Autodesk Fusion 360 part; units mm, degrees
sketch "base" plane through (0, 0, 0) normal (0, 0, 1) x (1, 0, 0)
  line L0 (0, 0) -> (19, 0)
  line L1 (19, 0) -> (19, 44.4)
  line L2 (19, 44.4) -> (0, 44.4)
  line L3 (0, 44.4) -> (0, 0)
  dimension "d1" = 19
  dimension "d2" = 44.4
extrude "Extrude1" add sketch "base" along normal blind 2
sketch "walls" plane through (0, 0, 2) normal (0, 0, 1) x (-1, 0, 0)
  line L0 (0, -44.4) -> (0, 0)
  line L1 (0, 0) -> (-19, 0)
  line L2 (-19, 0) -> (-19, -44.4)
  line L3 (-19, -44.4) -> (0, -44.4)
  line L4 (0, 0) -> (-19, 0)
  line L5 (-19, 0) -> (-19, -44.4)
  line L6 (-19, -44.4) -> (0, -44.4)
  line L7 (0, -44.4) -> (0, 0)
  line L8 (-1.2, -12) -> (-17.8, -12)
  line L9 (-17.8, -12) -> (-17.8, -36.4)
  line L10 (-15.3, -41.2) -> (-3.7, -41.2)
  line L11 (-1.2, -36.4) -> (-1.2, -12)
  line L12 (-1.2, -36.4) -> (-3.7, -41.2)
  line L13 (-17.8, -36.4) -> (-15.3, -41.2)
  dimension "d5" = 19
  dimension "d6" = 44.4
  dimension "d7" = 16.6
  dimension "d9" = 12
  dimension "d10" = 1.2
  dimension "d59" = 4.8
  dimension "d61" = 4.8
  dimension "d62" = 2.5
  dimension "d63" = 11.6
  dimension "d64" = 3.2
  dimension "d71" = 2.5
extrude "Extrude2" add sketch "walls" along normal blind 12
sketch "hole for connector" plane through (0, 0, 0) normal (0, -1, 0) x (1, 0, 0)
  line L0 (0, 0) -> (19, 0)
  line L1 (19, 0) -> (19, 14)
  line L2 (19, 14) -> (0, 14)
  line L3 (0, 14) -> (0, 0)
  line L4 (0, 14) -> (19, 14) construction
  line L5 (19, 14) -> (19, 2) construction
  line L6 (19, 2) -> (0, 2) construction
  line L7 (0, 2) -> (0, 14) construction
  line L8 (9.5, 14) -> (9.5, 0) construction
  line L9 (4.5, 8.4) -> (14.5, 8.4)
  line L10 (14.5, 8.4) -> (14.5, 2)
  line L11 (14.5, 2) -> (4.5, 2)
  line L12 (4.5, 2) -> (4.5, 8.4)
  dimension "d13" = 10
  dimension "d14" = 6.4
  dimension "d15" = 2
  dimension "d16" = 4.5
extrude "Extrude3" cut sketch "hole for connector" against normal blind 7 contours L9 L10 L11 L12
sketch "stand for rare of pcb" plane through (0, 0, 2) normal (0, 0, 1) x (-1, 0, 0)
  line L0 (-1.2, -12) -> (-17.8, -12)
  line L1 (-17.8, -12) -> (-17.8, -36.4)
  line L2 (-15.3, -41.2) -> (-3.7, -41.2)
  line L3 (-1.2, -36.4) -> (-1.2, -12)
  line L4 (-7.7, -41.2) -> (-11.3, -41.2)
  line L5 (-11.3, -41.2) -> (-11.3, -27)
  line L6 (-11.3, -27) -> (-7.7, -27)
  line L7 (-7.7, -27) -> (-7.7, -41.2)
  line L8 (-17.8, -12) -> (-1.2, -12)
  line L9 (-17.8, -36.4) -> (-15.3, -41.2)
  line L10 (-3.7, -41.2) -> (-1.2, -36.4)
  dimension "d27" = 3.6
  dimension "d28" = 15
  dimension "d29" = 6.5
extrude "Extrude5" add sketch "stand for rare of pcb" along normal blind 9 contours L2 L4 L5 L6 L7
sketch "hole for connector pins" plane through (0, 7, 0) normal (0, -1, 0) x (1, 0, 0)
  line L0 (4.5, 2) -> (14.5, 2)
  line L1 (14.5, 2) -> (14.5, 8.4)
  line L2 (14.5, 8.4) -> (4.5, 8.4)
  line L3 (4.5, 8.4) -> (4.5, 2)
  line L4 (5.5, 7.6) -> (13.5, 7.6)
  line L5 (13.5, 7.6) -> (13.5, 2)
  line L6 (13.5, 2) -> (5.5, 2)
  line L7 (5.5, 2) -> (5.5, 7.6)
  dimension "d32" = 8
  dimension "d33" = 5.6
  dimension "d34" = 5.5
  dimension "d35" = 2
extrude "Extrude6" cut sketch "hole for connector pins" against normal blind 5 contours L0 L4 L5 L6 L7
sketch "pit for pcb" plane through (0, 0, 14) normal (0, 0, 1) x (-1, 0, 0)
  line L0 (-1.2, -12) -> (-1.2, -36.4)
  line L1 (-3.7, -41.2) -> (-15.3, -41.2)
  line L2 (-17.8, -36.4) -> (-17.8, -12)
  line L3 (-17.8, -12) -> (-1.2, -12)
  line L4 (0, -44.4) -> (0, 0)
  line L5 (0, 0) -> (-19, 0)
  line L6 (-19, 0) -> (-19, -44.4)
  line L7 (-19, -44.4) -> (0, -44.4)
  line L8 (-2, -12) -> (-17, -12)
  line L9 (-17, -12) -> (-17, -3.2)
  line L10 (-17, -3.2) -> (-2, -3.2)
  line L11 (-2, -3.2) -> (-2, -12)
  line L12 (-1.2, -36.4) -> (-3.7, -41.2)
  line L13 (-15.3, -41.2) -> (-17.8, -36.4)
  dimension "d44" = 15
  dimension "d45" = 8.8
  dimension "d46" = 2
  dimension "d47" = 3.2
extrude "Extrude7" cut sketch "pit for pcb" against normal blind 3 contours L3 L8 L9 L10 L11
fillet "Fillet1" radius 1.5 4 edges at (19, 0, 7) (0, 0, 7) (0, 44.4, 7) (19, 44.4, 7)
sketch "pit for wires" plane through (0, 0, 11) normal (0, 0, 1) x (-1, 0, 0)
  line L0 (-2, -3.2) -> (-17, -3.2)
  line L1 (-17, -3.2) -> (-17, -12)
  line L2 (-2, -12) -> (-2, -3.2)
  line L3 (-4.5, -3.2) -> (-14.5, -3.2)
  line L4 (-14.5, -3.2) -> (-14.5, -7.2)
  line L5 (-4.5, -7.2) -> (-4.5, -3.2)
  line L6 (-2, -12) -> (-17, -12)
  line L7 (-17, -12) -> (-17, -7.2)
  line L8 (-2, -7.2) -> (-2, -12)
  line L9 (-17, -7.2) -> (-14.5, -7.2)
  line L10 (-4.5, -7.2) -> (-2, -7.2)
  line L11 (-17, -12) -> (-2, -12)
  dimension "d48" = 10
  dimension "d49" = 2.5
  dimension "d51" = 4
  dimension "d65" = 2.5
extrude "Extrude8" cut sketch "pit for wires" against normal blind 2 contours L0 L1 L2 L3 L4 L5 L6 L7 L8 L9 L10 L11
sketch "mount cylinder" plane through (0, 0, 11) normal (0, 0, 1) x (-1, 0, 0)
  line L0 (-7.7, -27) -> (-11.3, -27)
  line L1 (-11.3, -27) -> (-11.3, -41.2)
  line L2 (-11.3, -41.2) -> (-7.7, -41.2)
  line L3 (-7.7, -41.2) -> (-7.7, -27)
  circle A0 centre (-9.5, -38.2) radius 1
  line L4 (-17.8, -36.4) -> (-17.8, -12)
  dimension "d54" = 2
  dimension "d55" = 3
  dimension "d56" = 8.3
extrude "Extrude9" add sketch "mount cylinder" along normal blind 3 contours A0
sketch "mount cylinder 2" plane through (0, 0, 9) normal (0, 0, 1) x (-1, 0, 0)
  line L0 (-14.5, -3.2) -> (-14.5, -7.2)
  line L1 (-14.5, -7.2) -> (-17, -7.2)
  line L2 (-17, -7.2) -> (-17, -12)
  line L3 (-17, -12) -> (-2, -12)
  line L4 (-2, -12) -> (-2, -7.2)
  line L5 (-2, -7.2) -> (-4.5, -7.2)
  line L6 (-4.5, -7.2) -> (-4.5, -3.2)
  circle A0 centre (-9.5, -10.2) radius 1
  line L7 (-4.5, -3.2) -> (-14.5, -3.2)
  dimension "d66" = 2
  dimension "d68" = 7.5
  dimension "d72" = 7
extrude "Extrude10" add sketch "mount cylinder 2" along normal blind 3 contours A0
sketch "lock notch front" plane through (0, 0, 0) normal (0, -1, 0) x (1, 0, 0)
  line L0 (14.5, 8.4) -> (14.5, 2)
  line L1 (14.5, 2) -> (4.5, 2)
  line L2 (4.5, 2) -> (4.5, 8.4)
  line L3 (4.5, 8.4) -> (14.5, 8.4)
  line L4 (1.5, 14) -> (1.5, 0)
  line L5 (1.5, 0) -> (17.5, 0)
  line L6 (17.5, 0) -> (17.5, 14)
  line L7 (17.5, 14) -> (1.5, 14)
  line L8 (4.5, 12) -> (14.5, 12)
  line L9 (14.5, 12) -> (14.5, 10)
  line L10 (14.5, 10) -> (4.5, 10)
  line L11 (4.5, 10) -> (4.5, 12)
  dimension "d81" = 10
  dimension "d82" = 2
  dimension "d83" = 2
  dimension "d84" = 4.5
sketch "lock notch back" plane through (0, 44.4, 0) normal (0, 1, 0) x (-1, 0, 0)
  line L0 (-17.5, 14) -> (-17.5, 0)
  line L1 (-17.5, 0) -> (-1.5, 0)
  line L2 (-1.5, 0) -> (-1.5, 14)
  line L3 (-1.5, 14) -> (-17.5, 14)
  line L4 (-14.5, 12) -> (-4.5, 12)
  line L5 (-4.5, 12) -> (-4.5, 10)
  line L6 (-4.5, 10) -> (-14.5, 10)
  line L7 (-14.5, 10) -> (-14.5, 12)
  dimension "d85" = 10
  dimension "d86" = 2
  dimension "d87" = 2
  dimension "d88" = 4.5
extrude "Extrude12" cut sketch "lock notch back" against normal blind 2 contours L4 L5 L6 L7
extrude "Extrude13" cut sketch "lock notch front" against normal blind 2 contours L8 L9 L10 L11
fillet "Fillet2" radius 1 1 faces at (6.3333, 29.1, 0)
Verification items for the finished model (mm, model axes). A direction names the side the tool comes from. Round coordinates to 2 decimals unless told otherwise and drop trailing zeros. Order: outer loops, then holes, each group sorted by start corner. A loop starts at its lowest first (then second) coordinate and runs counter-clockwise, first axis right, second up. Notation, with made-up numbers: (66, -19.75) - (118, -19.75) arc R31 cw to (118, 14.25) - close; hole circle Ø9 at (79.25, 52). An arc over 180 degrees is marked (long way). Use CSV: the item, a comma, the result in double quotes. Start each with the question number.
1) Mould release check, pull along Y, two halves, no side actions. Record for faces 1 (the flat face through (4.5, 5, 10)), 2 (the flat face through (10, 38, 14)), 3 (the flat face through (9, 7, 8)), 4 (the flat face through (7.7, 34, 6)): +Y half, -Y half, draft (parallel to the pull), parting line (faces both ways), or undercut.
2) Thickness scan on L1, parallel to Y at x = 12.25, z = 12.25; L2, parallel to X at y = 14.5, z = 8.75; L3, parallel to X at y = 30, z = 8.75. Record the ranges inside material, lowest first.
3) Go/stop test with flat-tipped pins: P1, Ø8, axis at x = 6, y = 19.5, coming from the -Z side; P2, Ø2, axis at x = 10.5, y = 22.5, coming from the +Z side; P3, Ø3, axis at x = 10, z = 4.5, coming from the -Y side; P4, Ø2, axis at x = 10, y = 10, coming from the +Z side. Record where each tip stops, or that it passes through.
4) Section check A-A, the plane z = 13. Record the cut outline in (x, y).
5) Section check D-D, the plane y = 33. Record the cut outline in (x, z).
6) Access from +Z, -Z, +X, -X, +Y, -Y to the whole of each face (thin tool, end or side, straight path). Record for faces 5 (the flat face through (10, 34, 11)), 6 (the cylindrical face through (0.285, 21.91, 0.301)), 7 (the flat face through (4.5, 1, 11)).
7) Section check B-B, the plane x = 12.25. Record the cut outline in (y, z).
8) Section check C-C, the plane y = 5. Record the cut outline in (x, z).
Answers:
1,face 1,"undercut"
1,face 2,"draft"
1,face 3,"-Y half"
1,face 4,"undercut"
2,L1,"y = 0 to 3.2, 41.2 to 44.4"
2,L2,"x = 0 to 1.2, 17.8 to 19"
2,L3,"x = 0 to 1.2, 7.7 to 11.3, 17.8 to 19"
3,P1,"stops at z = 0"
3,P2,"stops at z = 2"
3,P3,"stops at y = 27"
3,P4,"stops at z = 12"
4,outline,"(0, 1.5) arc R1.5 ccw to (1.5, 0) - (17.5, 0) arc R1.5 ccw to (19, 1.5) - (19, 42.9) arc R1.5 ccw to (17.5, 44.4) - (1.5, 44.4) arc R1.5 ccw to (0, 42.9) - close; circle Ø2 at (9.5, 38.2); hole (1.2, 12) - (2, 12) - (2, 3.2) - (17, 3.2) - (17, 12) - (17.8, 12) - (17.8, 36.4) - (15.3, 41.2) - (3.7, 41.2) - (1.2, 36.4) - close"
5,outline,"(0, 1) arc R1 ccw to (1, 0) - (18, 0) arc R1 ccw to (19, 1) - (19, 14) - (17.8, 14) - (17.8, 2) - (11.3, 2) - (11.3, 11) - (7.7, 11) - (7.7, 2) - (1.2, 2) - (1.2, 14) - (0, 14) - close"
6,face 5,"+Z"
6,face 6,"-Z, -X, +Y, -Y"
6,face 7,"-Y"
7,outline,"(0, 1) arc R1 ccw to (1, 0) - (43.4, 0) arc R1 ccw to (44.4, 1) - (44.4, 10) - (42.4, 10) - (42.4, 12) - (44.4, 12) - (44.4, 14) - (41.2, 14) - (41.2, 2) - (0, 2) - close; (0, 8.4) - (7, 8.4) - (7, 7.6) - (12, 7.6) - (12, 9) - (3.2, 9) - (3.2, 14) - (0, 14) - (0, 12) - (2, 12) - (2, 10) - (0, 10) - close"
8,outline,"(0, 1) arc R1 ccw to (1, 0) - (18, 0) arc R1 ccw to (19, 1) - (19, 14) - (17, 14) - (17, 11) - (14.5, 11) - (14.5, 9) - (4.5, 9) - (4.5, 11) - (2, 11) - (2, 14) - (0, 14) - close; hole (4.5, 2) - (14.5, 2) - (14.5, 8.4) - (4.5, 8.4) - close"
